from build123d import *

# Parameters (mm, degrees)
F1_DEPTH = 30


with BuildPart() as f1:
    # F0 (on Top) → F1 (new body)
    with BuildSketch(Plane.XY):
        with BuildLine():
            ThreePointArc((34.478903, -20.278196), (19.860415, -34.721231), (0, -40))
            ThreePointArc((0, -40), (-20.139261, -34.56024), (-34.800884, -19.720508))
            Line((-34.800884, -19.720508), (-9.376239, -88.291404))
            ThreePointArc((-9.376239, -88.291404), (0.00745, -94.814889), (9.381409, -88.277428))
            Line((9.381409, -88.277428), (34.478903, -20.278196))
        make_face()
        with BuildLine():
            ThreePointArc((5, -84.814891), (0, -89.814891), (-5, -84.814891))
            Line((-5, -84.814891), (-5, -58.885846))
            ThreePointArc((-5, -58.885846), (0, -53.885846), (5, -58.885846))
            Line((5, -58.885846), (5, -84.814891))
        make_face(mode=Mode.SUBTRACT)
        with BuildLine():
            ThreePointArc((0, 20), (14.142136, 14.142136), (20, 0))
            ThreePointArc((20, 0), (14.142136, -14.142136), (0, -20))
            Line((0, -20), (0, -40))
            ThreePointArc((0, -40), (19.860415, -34.721231), (34.478903, -20.278196))
            ThreePointArc((34.478903, -20.278196), (38.595052, -10.508184), (40, 0))
            ThreePointArc((40, 0), (28.284271, 28.284271), (0, 40))
            Line((0, 40), (0, 20))
        make_face()
        with BuildLine():
            ThreePointArc((0, -20), (-20, 0), (0, 20))
            Line((0, 20), (0, 40))
            ThreePointArc((0, 40), (-34.56024, 20.139261), (-34.800884, -19.720508))
            ThreePointArc((-34.800884, -19.720508), (-20.139261, -34.56024), (0, -40))
            Line((0, -40), (0, -20))
        make_face()
        with BuildLine():
            ThreePointArc((-34.800884, -19.720508), (-34.56024, 20.139261), (0, 40))
            Line((0, 40), (-75.554794, 55.409922))
            ThreePointArc((-75.554794, 55.409922), (-86.170881, 50.684701), (-85.150626, 39.109378))
            Line((-85.150626, 39.109378), (-34.800884, -19.720508))
        make_face()
        with BuildLine():
            ThreePointArc((-79.551648, 41.02838), (-82.136483, 47.610069), (-75.554794, 50.194904))
            Line((-75.554794, 50.194904), (-59.814075, 43.331522))
            ThreePointArc((-59.814075, 43.331522), (-57.22924, 36.749833), (-63.810929, 34.164998))
            Line((-63.810929, 34.164998), (-79.551648, 41.02838))
        make_face(mode=Mode.SUBTRACT)
        with BuildLine():
            Line((77.689324, 54.912919), (0, 40))
            ThreePointArc((0, 40), (28.284271, 28.284271), (40, 0))
            ThreePointArc((40, 0), (38.595052, -10.508184), (34.478903, -20.278196))
            Line((34.478903, -20.278196), (87.025319, 38.422523))
            ThreePointArc((87.025319, 38.422523), (88.276625, 50.018919), (77.689324, 54.912919))
        make_face()
        with BuildLine():
            ThreePointArc((76.795383, 49.248739), (83.73099, 47.871297), (82.353549, 40.935689))
            Line((82.353549, 40.935689), (61.591367, 27.053942))
            ThreePointArc((61.591367, 27.053942), (54.655759, 28.431383), (56.033201, 35.366991))
            Line((56.033201, 35.366991), (76.795383, 49.248739))
        make_face(mode=Mode.SUBTRACT)
    extrude(amount=F1_DEPTH)


solid = f1.part
Can you work these out from the model? Positions are in its coordinate system, mm. A direction names the side the tool comes from. Round coordinates to 2 decimals unless told otherwise and drop trailing zeros. Loops run counter-clockwise (first coordinate to the right, second up) from the corner with the lowest first, then second, coordinate; pieces in that order, holes last. Notation, with made-up numbers: (29.25, 22.25) - (50.25, 22.25) arc R23 ccw to (50.25, 48.25) - close; hole circle Ø9 at (2.5, -14.75). An arc over 180 degrees is marked (long way). Answer in a Markdown table with one row per item. Add a question column.
Q1. I want a section at C-C on x = 64.5. List the corners of the cut face in (y, z) for me.
Q2. I want a section at B-B on y = -77. List the corners of the cut face in (x, z) for me, and give its area (3 significant figures).
Q3. For pin 1 Ø4 at (y, z) = (23, 10.5) entering from -X; pin 2 Ø10 at (x, z) = (-39.5, 19.5) entering from +Y; pin 3 Ø1 at (y, z) = (-10.5, 23) entering from +X, each with a flat end and sliding along its axis, tell me the tip position at first contact or that it passes through.
Q4. I need wall thicknesses on L1, parallel to Y at x = -1, z = 25; L2, parallel to Y at x = 66, z = 4.75; L3, parallel to X at y = -79.5, z = 4.25. Which ranges of each line are inside material? Lowest first, please.
Q5. I want a section at D-D on y = -46. List the corners of the cut face in (x, z) for me.
Q6. We'd pull the mould along X, two halves only. Please class faces 4 (the flat face through (-71.57, 37.55, 14.79)), 5 (the flat face through (-60.33, 10.11, 14.79)), 6 (the cylindrical face through (-0.163, -94.814, 14.79)): pulls with the +X half, pulls with the -X half, needs draft (parallel to the pull), parting line crosses it, or undercut.
Q7. Which directions (+Z, -Z, +X, -X, +Y, -Y) give clear straight access to the entire face, cutting with the end or side of a thin tool? Please do faces 1 (the cylindrical face through (-0.11, -53.887, 14.79)), 2 (the flat face through (60.384, 8.661, 14.79)), 3 (the flat face through (-37.249, 47.597, 14.79)).
Q8. I want a section at A-A on z = 12. List the corners of the cut face in (x, y) for me (1 decimal).
A:
| question | item | result |
|---|---|---|
| 1 | outline | (13.26, 0) - (29, 0) - (29, 30) - (13.26, 30) - close; (41.03, 0) - (52.38, 0) - (52.38, 30) - (41.03, 30) - close |
| 2 | outline | (-13.56, 0) - (-5, 0) - (-5, 30) - (-13.56, 30) - close; (5, 0) - (13.54, 0) - (13.54, 30) - (5, 30) - close |
| 2 | area | 513 mm^2 |
| 3 | pin 1 | x = -73.08 |
| 3 | pin 2 | y = 49.08 |
| 3 | pin 3 | x = 43.68 |
| 4 | L1 | -94.76 to -89.71, -53.99 to -19.97, 19.97 to 40.2 |
| 4 | L2 | 14.93 to 30, 42.03 to 52.67 |
| 4 | L3 | -12.64 to -5, 5 to 12.62 |
| 5 | outline | (-25.06, 0) - (24.99, 0) - (24.99, 30) - (-25.06, 30) - close |
| 6 | face 4 | undercut |
| 6 | face 5 | pulls with the -X half |
| 6 | face 6 | parting line crosses it |
| 7 | face 1 | +Z, -Z |
| 7 | face 2 | +Z, -Z, +X, -Y |
| 7 | face 3 | +Z, -Z, +Y |
| 8 | outline | (-85.2, 39.1) - (-34.8, -19.7) - (-9.4, -88.3) arc R10 ccw to (9.4, -88.3) - (34.5, -20.3) - (87, 38.4) arc R10 ccw to (77.7, 54.9) - (0, 40) - (-75.6, 55.4) arc R10 ccw to start; hole (-79.6, 41) - (-63.8, 34.2) arc R5 ccw to (-59.8, 43.3) - (-75.6, 50.2) arc R5 ccw to start; hole (-5, -84.8) arc R5 ccw to (5, -84.8) - (5, -58.9) arc R5 ccw to (-5, -58.9) - close; hole (0, -20) arc R20 ccw to (20, 0) arc R20 ccw to (0, 20) arc R20 ccw to start; hole (56, 35.4) arc R5 ccw to (61.6, 27.1) - (82.4, 40.9) arc R5 ccw to (76.8, 49.2) - close |
